from build123d import *

# Parameters (mm, degrees)
F0_R     = 3.2385
F1_DEPTH = 3.175


with BuildPart() as f1:
    # F0 (on Top) → F1 (new body)
    with BuildSketch(Plane.XY):
        with BuildLine():
            ThreePointArc((0, 6.35), (1.859872, 1.859872), (6.35, 0))
            Line((6.35, 0), (44.45, 0))
            ThreePointArc((44.45, 0), (48.940128, 1.859872), (50.8, 6.35))
            Line((50.8, 6.35), (50.8, 171.45))
            ThreePointArc((50.8, 171.45), (48.940128, 175.940128), (44.45, 177.8))
            Line((44.45, 177.8), (6.35, 177.8))
            ThreePointArc((6.35, 177.8), (1.859872, 175.940128), (0, 171.45))
            Line((0, 171.45), (0, 6.35))
        make_face()
        with Locations((38.1, 12.7)):
            Circle(F0_R, mode=Mode.SUBTRACT)
        with Locations((38.1, 25.4)):
            Circle(F0_R, mode=Mode.SUBTRACT)
        with Locations((38.1, 38.1)):
            Circle(F0_R, mode=Mode.SUBTRACT)
        with Locations((38.1, 50.8)):
            Circle(F0_R, mode=Mode.SUBTRACT)
        with Locations((38.1, 63.5)):
            Circle(F0_R, mode=Mode.SUBTRACT)
        with Locations((38.1, 76.2)):
            Circle(F0_R, mode=Mode.SUBTRACT)
        with Locations((38.1, 88.9)):
            Circle(F0_R, mode=Mode.SUBTRACT)
        with Locations((38.1, 101.6)):
            Circle(F0_R, mode=Mode.SUBTRACT)
        with Locations((38.1, 114.3)):
            Circle(F0_R, mode=Mode.SUBTRACT)
        with Locations((38.1, 127)):
            Circle(F0_R, mode=Mode.SUBTRACT)
        with Locations((38.1, 139.7)):
            Circle(F0_R, mode=Mode.SUBTRACT)
        with Locations((38.1, 152.4)):
            Circle(F0_R, mode=Mode.SUBTRACT)
        with Locations((38.1, 165.1)):
            Circle(F0_R, mode=Mode.SUBTRACT)
    extrude(amount=F1_DEPTH)


solid = f1.part
Geometry check sheet. Reference: the model listing, model coordinates, mm. Give positions to 0.01 mm unless a question says otherwise; leave off trailing zeros. Loops run counter-clockwise (first coordinate to the right, second up) from the corner with the lowest first, then second, coordinate; pieces in that order, holes last.
(1) Section check A-A on y = 139.7. Record the cut outline in (x, z) (1 decimal).
From the geometry:
outline: (0, 0) - (34.9, 0) - (34.9, 3.2) - (0, 3.2) - close; (41.3, 0) - (50.8, 0) - (50.8, 3.2) - (41.3, 3.2) - close
(2) Section check B-B on z = 1.35. Count the separate pieces of the cut face and the enclosed holes in it, then the cut area to 3 significant figures.
From the geometry:
separate pieces: 1
enclosed holes: 13
area: 8,570 mm2
(3) Thickness scan on L1, parallel to X at y = 152.4, z = 1.15; L2, parallel to X at y = 49.5, z = 1.6; L3, parallel to Y at x = 3, z = 1.1. Record the ranges inside material, lowest first.
From the geometry:
L1: x = 0 to 34.86, 41.34 to 50.8
L2: x = 0 to 35.13, 41.07 to 50.8
L3: y = 0.96 to 176.84
(4) Release check for a two-part mould opening along Y. For faces 1 (the cylindrical face through (41.19, 115.27, 1.57)), 2 (the flat face through (50.8, 88, 2)), 3 (the cylindrical face through (48.89, 1.81, 1.57)), 4 (the flat face through (26, 177.8, 2)) record: released by +Y, released by -Y, zero draft, split by the parting line, or undercut.
From the geometry:
face 1: undercut
face 2: zero draft
face 3: released by -Y
face 4: released by +Y
